```python
from build123d import *

# Parameters (mm, degrees)
EXTRUDE_1_DEPTH      = 10
EXTRUDE_3_DEPTH      = 4
EXTRUDE_3_DEPTH_BACK = 4
FILLET_3_R           = 1
CUT_EXTRUDE_2_DEPTH  = 1


with BuildPart() as part:
    # 草图1 → 凸台-拉伸1 (new body)
    with BuildSketch(Plane.XY):
        Polygon((0, 0), (0, 2.5), (11, 2.5), (11, 0), (13, 0), (13, 4.5), (-2, 4.5), (-2, 0), align=None)
    extrude(amount=EXTRUDE_1_DEPTH)

    # 草图7 → 凸台-拉伸3 (add, two sides: drawn at the far end of the back side and taken through both)
    with BuildSketch(Plane(origin=(5.5, 0, 0), x_dir=(0, 0, -1), z_dir=(1, 0, 0)).offset(-EXTRUDE_3_DEPTH_BACK)):
        Polygon((-9, 4.5), (-5, 19.5), (-1, 4.5), align=None)
    extrude(amount=EXTRUDE_3_DEPTH + EXTRUDE_3_DEPTH_BACK)

    # 圆角3
    fillet_3_edges = [part.edges().sort_by_distance(p)[0] for p in [
        (5.5, 4.5, 1),
        (5.5, 4.5, 9),
        (5.5, 19.5, 5),
    ]]
    fillet(fillet_3_edges, radius=FILLET_3_R)

    # 草图8 → 切除-拉伸2 (cut)
    with BuildSketch(Plane(origin=(9.5, 0, 0), x_dir=(0, 0, -1), z_dir=(1, 0, 0))):
        with BuildLine():
            Line((-2.636988353, 6.757662651), (-4.03376506, 11.995575302))
            ThreePointArc((-4.03376506, 11.995575302), (-5, 12.737912652), (-5.96623494, 11.995575302))
            Line((-5.96623494, 11.995575302), (-7.363011647, 6.757662651))
            ThreePointArc((-7.363011647, 6.757662651), (-7.189765563, 5.89076386), (-6.396776707, 5.5))
            Line((-6.396776707, 5.5), (-3.603223293, 5.5))
            ThreePointArc((-3.603223293, 5.5), (-2.810234437, 5.89076386), (-2.636988353, 6.757662651))
        make_face()
        with BuildLine():
            ThreePointArc((-6.879894177, 6.628831325), (-6.793271135, 6.19538193), (-6.396776707, 6))
            Line((-6.396776707, 6), (-3.603223293, 6))
            ThreePointArc((-3.603223293, 6), (-3.206728865, 6.19538193), (-3.120105823, 6.628831325))
            Line((-3.120105823, 6.628831325), (-4.51688253, 11.866743977))
            ThreePointArc((-4.51688253, 11.866743977), (-5, 12.237912652), (-5.48311747, 11.866743977))
            Line((-5.48311747, 11.866743977), (-6.879894177, 6.628831325))
        make_face(mode=Mode.SUBTRACT)
    cut_extrude_2 = extrude(amount=-CUT_EXTRUDE_2_DEPTH, mode=Mode.SUBTRACT)

    # 镜向1: 切除-拉伸2 across plane
    add(cut_extrude_2.mirror(Plane(origin=(5.5, 0, 0), x_dir=(0, 0, 1), z_dir=(1, 0, 0))), mode=Mode.SUBTRACT)


solid = part.part
```
Input: part model. Units: mm. Frame: model coordinates. A direction names the side the tool comes from. Give positions to 0.01 mm unless a question says otherwise; leave off trailing zeros. Order: outer loops, then holes, each group sorted by start corner. A loop starts at its lowest first (then second) coordinate and runs counter-clockwise, first axis right, second up. Notation, with made-up numbers: (39, -32) -> (64, -32) arc R23 cw to (64, -14) -> close; hole circle Ø11 at (87.5, -13). An arc over 180 degrees is marked (long way). Write each question's results on one line, items separated by ' | '. Start each with the question number.
Item 1: Cut plane C-C on x = 5. Return the cut outline in (y, z), then the cut area to 3 significant figures.
Item 2: Cut plane A-A on y = 2. Return the cut outline in (x, z), then the cut area to 3 significant figures.
Item 3: Cut plane B-B on z = 2. Return the cut outline in (x, y), then the cut area to 3 significant figures.
Item 4: Set-up query: faces 4 (the flat face through (11, 1, 5)), 5 (the flat face through (2, 6, 5)), 6 (the flat face through (8.5, 8.3, 6.6)). Return all of +Z, -Z, +X, -X, +Y, -Y with unobstructed straight access to the full face (end or side cutting, diameter ignored); none if empty.
Item 5: Cut plane D-D on z = 5. Return the cut outline in (x, y).
Item 6: Line query: line 1 (X direction, y = 1.75, z = 5.5); line 2 (X direction, y = 6.5, z = 7); line 3 (X direction, y = 13.25, z = 6.25). Output: solid intervals per line, ascending.
Item 7: Contact query for flat-ended pins moving along their axis: P1, Ø0.5, axis at x = 2, z = 5, coming from the -Y side; P2, Ø0.8, axis at x = 9, z = 4.5, coming from the +Y side; P3, Ø4, axis at y = 7, z = 2.5, coming from the +X side. Output: stop coordinate, or through.
Item 8: Mould query, pull axis Z, two halves, no side actions, for faces 1 (the cylindrical face through (1.993, 12.238, 4.991)), 2 (the flat face through (1.5, 8, 5)), 3 (the cylindrical face through (5.56, 16.62, 4.98)). Classes: pulls with the +Z half, pulls with the -Z half, needs draft (parallel to the pull), parting line crosses it, or undercut.
Established:
1) outline: (2.5, 0) -> (4.5, 0) -> (4.5, 0.23) arc R1 cw to (5.24, 1.2) -> (15.88, 4.03) arc R1 ccw to (15.88, 5.97) -> (5.24, 8.8) arc R1 cw to (4.5, 9.77) -> (4.5, 10) -> (2.5, 10) -> close | area: 77.8 mm^2
2) outline: (-2, 0) -> (0, 0) -> (0, 10) -> (-2, 10) -> close; (11, 0) -> (13, 0) -> (13, 10) -> (11, 10) -> close | area: 40.0 mm^2
3) outline: (-2, 0) -> (0, 0) -> (0, 2.5) -> (11, 2.5) -> (11, 0) -> (13, 0) -> (13, 4.5) -> (9.5, 4.5) -> (9.5, 8.25) -> (1.5, 8.25) -> (1.5, 4.5) -> (-2, 4.5) -> close | area: 70.0 mm^2
4) face 4: +Z, -Z, -Y | face 5: -X | face 6: +X
5) outline: (-2, 0) -> (0, 0) -> (0, 2.5) -> (11, 2.5) -> (11, 0) -> (13, 0) -> (13, 4.5) -> (9.5, 4.5) -> (9.5, 5.5) -> (8.5, 5.5) -> (8.5, 6) -> (9.5, 6) -> (9.5, 12.24) -> (8.5, 12.24) -> (8.5, 12.74) -> (9.5, 12.74) -> (9.5, 16.62) -> (1.5, 16.62) -> (1.5, 12.74) -> (2.5, 12.74) -> (2.5, 12.24) -> (1.5, 12.24) -> (1.5, 6) -> (2.5, 6) -> (2.5, 5.5) -> (1.5, 5.5) -> (1.5, 4.5) -> (-2, 4.5) -> close
6) line 1: -2 to 0, 11 to 13 | line 2: 2.5 to 8.5 | line 3: 1.5 to 9.5
7) P1: y = 2.5 | P2: y = 16.61 | P3: x = 9.5
8) face 1: undercut | face 2: needs draft | face 3: parting line crosses it
